Check sheet for the modelled part. Datum: model origin and axes. Units: mm. Face numbers are marked on the shaded views. A direction names the side the tool comes from. Round coordinates to 2 decimals unless told otherwise and drop trailing zeros. Write each loop counter-clockwise with the first axis right and the second up, starting at its lowest first coordinate (ties: lowest second). Pieces come first, ordered by that corner, then holes. Notation, with made-up numbers: M 58,-12.5 L 64,-12.5 A28 ccw 64,16.5 Z; hole C 55.5,28.5 d7. An arc over 180 degrees is marked long. Put each result on its own line as item: value.
```python
from build123d import *

# Parameters (mm, degrees)
F0_R     = 10.915306
F1_DEPTH = 18.8


with BuildPart() as f1:
    # F0 (on Front) → F1 (new body)
    with BuildSketch(Plane.XZ):
        Polygon((-8.224501, -18.871788), (-14.783561, -18.871788), (-14.783561, -25.250662), (-14.783561, -40.478557), (-14.783561, -46.743103), (-8.224501, -46.743103), (8.224501, -46.743103), (14.783561, -46.743103), (14.783561, -40.478557), (14.783561, -25.230598), (14.783561, -18.871788), (8.224771, -18.871788), align=None)
        with Locations((0, -32.807445)):
            Circle(F0_R, mode=Mode.SUBTRACT)
        with BuildLine():
            Line((-16.529163, 10.306755), (-8.224501, -18.871788))
            Line((-8.224501, -18.871788), (8.224771, -18.871788))
            Line((8.224771, -18.871788), (16.306807, 10.15533))
            ThreePointArc((16.306807, 10.15533), (10.12712, 9.707231), (6.4558, 14.698296))
            Line((6.4558, 14.698296), (0, 12.95887))
            Line((0, 12.95887), (-6.4558, 14.698296))
            ThreePointArc((-6.4558, 14.698296), (-10.249858, 9.652182), (-16.529163, 10.306755))
        make_face()
        Polygon((9.45, -5.361695), (0, -10.817656), (-9.45, -5.361695), (-9.45, 5.550225), (0, 11.006185), (9.45, 5.550225), align=None, mode=Mode.SUBTRACT)
        with BuildLine():
            Line((-14.783561, -40.478557), (-14.783561, -25.250662))
            Line((-14.783561, -25.250662), (-42.868647, -13.980851))
            ThreePointArc((-42.868647, -13.980851), (-41.905671, -19.987009), (-46.035767, -24.452832))
            Line((-46.035767, -24.452832), (-44.79609, -32.854578))
            Line((-44.79609, -32.854578), (-46.035767, -41.256323))
            ThreePointArc((-46.035767, -41.256323), (-41.900736, -45.738537), (-42.888374, -51.756284))
            Line((-42.888374, -51.756284), (-14.783561, -40.478557))
        make_face()
        Polygon((-32.240685, -43.477823), (-41.440685, -38.1662), (-41.440685, -27.542955), (-32.240685, -22.231333), (-23.040685, -27.542955), (-23.040685, -38.1662), align=None, mode=Mode.SUBTRACT)
        with BuildLine():
            Line((42.888374, -13.952871), (14.783561, -25.230598))
            Line((14.783561, -25.230598), (14.783561, -40.478557))
            Line((14.783561, -40.478557), (42.888374, -51.756284))
            ThreePointArc((42.888374, -51.756284), (41.900736, -45.738537), (46.035767, -41.256323))
            Line((46.035767, -41.256323), (44.79609, -32.854578))
            Line((44.79609, -32.854578), (46.035767, -24.452832))
            ThreePointArc((46.035767, -24.452832), (41.900736, -19.970619), (42.888374, -13.952871))
        make_face()
        Polygon((32.240685, -43.766498), (22.790685, -38.310538), (22.790685, -27.398618), (32.240685, -21.942658), (41.690685, -27.398618), (41.690685, -38.310538), align=None, mode=Mode.SUBTRACT)
        with BuildLine():
            Line((8.224501, -46.743103), (-8.224501, -46.743103))
            Line((-8.224501, -46.743103), (-16.529163, -75.921646))
            ThreePointArc((-16.529163, -75.921646), (-10.249858, -75.267073), (-6.4558, -80.313187))
            Line((-6.4558, -80.313187), (0, -78.573761))
            Line((0, -78.573761), (6.4558, -80.313187))
            ThreePointArc((6.4558, -80.313187), (10.249858, -75.267073), (16.529163, -75.921646))
            Line((16.529163, -75.921646), (8.224501, -46.743103))
        make_face()
        Polygon((-9.45, -71.165115), (-9.45, -60.253195), (0, -54.797235), (9.45, -60.253195), (9.45, -71.165115), (0, -76.621075), align=None, mode=Mode.SUBTRACT)
    extrude(amount=F1_DEPTH)


solid = f1.part
```
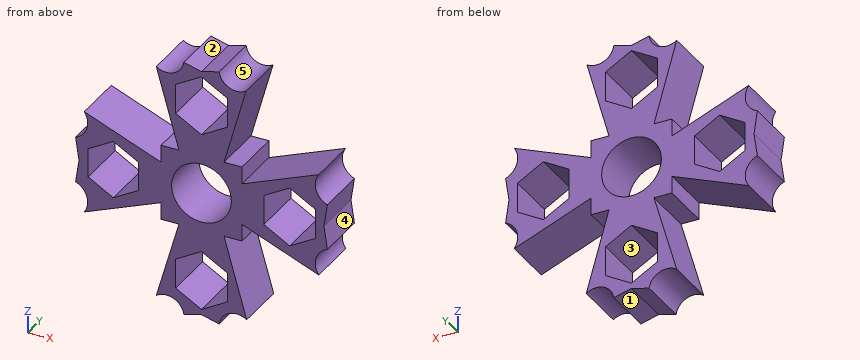
1. Cross-section at D-D (y = -16.5). Count the separate pieces of the cut face and the enclosed holes in it, then the cut area to 3 significant figures.
Computed values:
separate pieces: 1
enclosed holes: 5
area: 2,310 mm2
2. Depth check by flat-ended pin: pin 1 Ø2 at (x, y) = (-10.5, -9) entering from +Z; pin 2 Ø10 at (y, z) = (-9.5, -2.5) entering from -X; pin 3 Ø8.5 at (y, z) = (-6, -35) entering from -X. Enter the tip coordinate at first touch or a pass-through.
Computed values:
pin 1: stops at z = 10.04
pin 2: stops at x = -14.31
pin 3: stops at x = -45.74
3. Cross-section at B-B (x = 35). Enter the section's corners in (y, z).
Computed values:
outline: M -18.8,-48.59 L 0,-48.59 L 0,-42.17 L -18.8,-42.17 Z; M -18.8,-23.54 L 0,-23.54 L 0,-17.12 L -18.8,-17.12 Z
4. Cross-section at A-A (z = -58.5). Enter the section's corners in (x, y).
Computed values:
outline: M -11.57,-18.8 L -6.41,-18.8 L -6.41,0 L -11.57,0 Z; M 6.41,-18.8 L 11.57,-18.8 L 11.57,0 L 6.41,0 Z
5. Scan lines: probe 1 along Z at (x, y) = (0, -13.5); probe 2 along X at (y, z) = (-1.75, -46.5); probe 3 along X at (y, z) = (-17, -18.5). Record each from-to range of solid material in increasing order.
Computed values:
probe 1: z = -78.57 to -76.62, -54.8 to -43.72, -21.89 to -10.82, 11.01 to 12.96
probe 2: x = -41.72 to -29.79, -14.78 to 14.78, 29.79 to 41.72
probe 3: x = -41.63 to -31.61, -8.33 to 8.33, 31.56 to 41.63
6. Cross-section at C-C (z = -20.5). Enter the section's corners in (x, y), then the cut area to 3 significant figures.
Computed values:
outline: M -42.08,-18.8 L -26.62,-18.8 L -26.62,0 L -42.08,0 Z; M -14.78,-18.8 L 14.78,-18.8 L 14.78,0 L -14.78,0 Z; M 26.57,-18.8 L 42.08,-18.8 L 42.08,0 L 26.57,0 Z
area: 1,140 mm2
7. Release check for a two-part mould opening along X. For the marked faces 4 and 5 record: +X half, -X half, draft (parallel to the pull), parting line (faces both ways), or undercut.
Computed values:
face 4: +X half
face 5: undercut
8. Access from +Z, -Z, +X, -X, +Y, -Y to the whole of each face (thin tool, end or side, straight path). Record for the marked faces 1, 2 and 3.
Computed values:
face 1: -Z, +Y, -Y
face 2: +Z, +Y, -Y
face 3: +Y, -Y
